Geometry check sheet. Reference: the model listing, model coordinates, mm. A direction names the side the tool comes from. Give positions to 0.01 mm unless a question says otherwise; leave off trailing zeros. Order: outer loops, then holes, each group sorted by start corner. A loop starts at its lowest first (then second) coordinate and runs counter-clockwise, first axis right, second up. Notation, with made-up numbers: M -5,-7.5 L 15,-7.5 A23 cw 15,23.5 Z; hole C 15.5,60.25 d7. An arc over 180 degrees is marked long. Put each result on its own line as item: value. Start each with the question number.
Q1. Section check A-A on y = 0. Record the cut outline in (x, z), then the cut area to 3 significant figures.
Q2. Section check B-B on z = 14.5. Record the cut outline in (x, y), then the cut area to 3 significant figures.
Q3. Go/stop test with flat-tipped pins: pin 1 (3 mm diameter, centred on x = -2, y = 2, fed in from +Z); pin 2 (2 mm diameter, centred on x = 0, y = -0.5, fed in from -Z); pin 3 (1 mm diameter, centred on y = -2, z = 9, fed in from -X); pin 4 (1.5 mm diameter, centred on y = 2, z = 4.5, fed in from +X). Record where each tip stops, or that it passes through.
Q4. Mould release check, pull along Y, two halves, no side actions. Record for faces 1 (the cylindrical face through (-2.8, 0.1, 1.5)), 2 (the flat face through (1.298, -0.055, 1.113)), 3 (the flat face through (0, -2, 3)): +Y half, -Y half, draft (parallel to the pull), parting line (faces both ways), or undercut.
Q5. Access from +Z, -Z, +X, -X, +Y, -Y to the whole of each face (thin tool, end or side, straight path). Record for faces 4 (the cylindrical face through (-1.45, 0.06, 11.75)), 5 (the flat face through (0, 0, 21)), 6 (the flat face through (-0.697, -1.096, 1.113)).
Q6. Material ranges on L1, parallel to Z at x = 0.3, y = 1.7; L2, parallel to Z at x = 0.35, y = -0.45; L3, parallel to X at y = -0.1, z = 16.25, recorded low to high.
```python
from build123d import *

# Parameters (mm, degrees)
SKETCH_R     = 2.8
PAD_DEPTH    = 3
SKETCH001_R  = 1.45
PAD001_DEPTH = 18
POCKET_DEPTH = 2
CHAMFER_SIZE = 0.25


with BuildPart() as part:
    # Sketch → Pad (new body)
    with BuildSketch(Plane.XY):
        Circle(SKETCH_R)
    extrude(amount=PAD_DEPTH)

    # Sketch001 (on Face3 of Pad) → Pad001 (join)
    with BuildSketch(Plane.XY.offset(3)):
        Circle(SKETCH001_R)
    extrude(amount=PAD001_DEPTH)

    # Sketch002 (on Face2 of Pad001) → Pocket (cut)
    with BuildSketch(Plane(origin=(0, 0, 0), x_dir=(1, 0, 0), z_dir=(0, 0, -1))):
        Polygon((1.259542, 0.814588), (-0.075682, 1.49809), (-1.335225, 0.683502), (-1.259542, -0.814588), (0.075682, -1.49809), (1.335225, -0.683502), align=None)
    extrude(amount=-POCKET_DEPTH, mode=Mode.SUBTRACT)

    # Chamfer
    chamfer_edges = [part.edges().sort_by_distance(p)[0] for p in [
        (-2.8, 0, 3),
        (-2.8, 0, 0),
        (1.297384, -0.065543, 0),
        (0.705454, 1.090796, 0),
        (-0.59193, 1.156339, 0),
        (-1.297384, 0.065543, 0),
        (-0.705454, -1.090796, 0),
        (0.59193, -1.156339, 0),
        (-1.45, 0, 21),
    ]]
    chamfer(chamfer_edges, length=CHAMFER_SIZE)


solid = part.part
```
Results found:
1. outline: M -2.8,0.25 L -2.55,0 L -1.55,0 L -1.3,0.25 L -1.3,2 L 1.3,2 L 1.3,0.25 L 1.55,0 L 2.55,0 L 2.8,0.25 L 2.8,2.75 L 2.55,3 L 1.45,3 L 1.45,20.75 L 1.2,21 L -1.2,21 L -1.45,20.75 L -1.45,3 L -2.55,3 L -2.8,2.75 Z
1. area: 63.5 mm^2
2. outline: C 0,0 d2.9
2. area: 6.61 mm^2
3. pin 1: stops at z = 20.87
3. pin 2: stops at z = 0.1
3. pin 3: passes through
3. pin 4: stops at x = 0.73
4. face 1: parting line
4. face 2: undercut
4. face 3: draft
5. face 4: +Z
5. face 5: +Z, +X, -X, +Y, -Y
5. face 6: -Z
6. L1: z = 0 to 3
6. L2: z = 2 to 21
6. L3: x = -1.45 to 1.45
